from build123d import *

# Parameters (mm, degrees)
SKETCH1_W                  = 231.4
SKETCH1_H                  = 30
BOSS_EXTRUDE1_DEPTH        = 3
BOSS_EXTRUDE2_DEPTH        = 3
F_8_0_8_DIAMETER_HOLE1_D   = 8
F_8_0_8_DIAMETER_HOLE2_D   = 8
F_10_0_10_DIAMETER_HOLE1_D = 10


with BuildPart() as part:
    # Sketch1 → Boss-Extrude1 (new body)
    with BuildSketch(Plane.XY):
        with Locations((0, -15)):
            Rectangle(SKETCH1_W, SKETCH1_H)
    extrude(amount=BOSS_EXTRUDE1_DEPTH)

    # Sketch2 → Boss-Extrude2 (add)
    with BuildSketch(Plane(origin=(0, 0, 0), x_dir=(1, 0, 0), z_dir=(0, 1, 0))):
        Polygon((-115.7, -3), (115.7, -3), (85.7, -33), (-85.7, -33), align=None)
    extrude(amount=-BOSS_EXTRUDE2_DEPTH)

    # Ø8.0 (8) Diameter Hole1 (through all)
    with Locations(Plane.XY.offset(3)):
        with Locations((-100.7, -15), (100.7, -15)):
            Hole(F_8_0_8_DIAMETER_HOLE1_D / 2)

    # Ø8.0 (8) Diameter Hole2 (through all)
    with Locations(Plane(origin=(0, 0, 0), x_dir=(1, 0, 0), z_dir=(0, 1, 0))):
        with Locations((0, -18)):
            Hole(F_8_0_8_DIAMETER_HOLE2_D / 2)

    # Ø10.0 (10) Diameter Hole1 (through all)
    with Locations(Plane.XY.offset(3)):
        with Locations((62.5, -15)):
            Hole(F_10_0_10_DIAMETER_HOLE1_D / 2)


solid = part.part
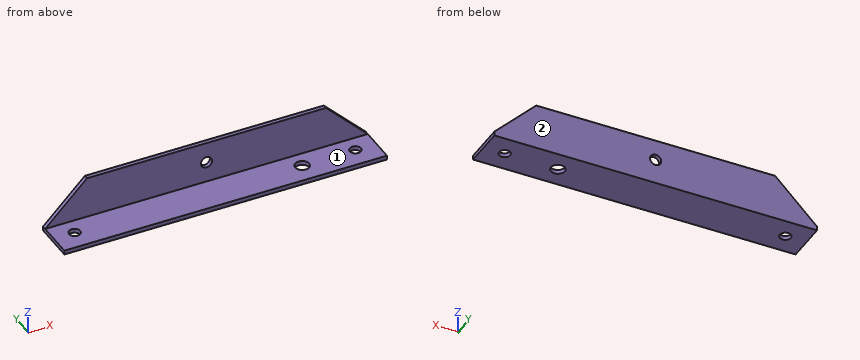
Here's how the part is built. I have some questions about the finished solid (model axes, mm). Face numbers are marked on the shaded views. A direction names the side the tool comes from. Coordinates: 2 decimals unless noted, no trailing zeros. Write each loop counter-clockwise with the first axis right and the second up, starting at its lowest first coordinate (ties: lowest second). Pieces come first, ordered by that corner, then holes.
1) I'm going to push flat-ended pins straight in: pin 1 (3 mm diameter, centred on x = -5.5, y = -16.5, fed in from +Z); pin 2 (10 mm diameter, centred on y = -10.5, z = 25.5, fed in from +X); pin 3 (15 mm diameter, centred on x = -5.5, z = 25.5, fed in from -Y). Where does each tip first touch, or does it pass through?
Filled in:
pin 1: stops at z = 3
pin 2: passes through
pin 3: stops at y = -3
2) If we section it at B-B (y = -15): List the corners of the cut face in (x, z) for me, plus the area to 3 significant figures.
Filled in:
outline: (-115.7, 0) - (-104.7, 0) - (-104.7, 3) - (-115.7, 3) - close; (-96.7, 0) - (57.5, 0) - (57.5, 3) - (-96.7, 3) - close; (67.5, 0) - (96.7, 0) - (96.7, 3) - (67.5, 3) - close; (104.7, 0) - (115.7, 0) - (115.7, 3) - (104.7, 3) - close
area: 616 mm2
3) If we section it at C-C (z = 18): List the corners of the cut face in (x, y) for me.
Filled in:
outline: (-100.7, -3) - (-4, -3) - (-4, 0) - (-100.7, 0) - close; (4, -3) - (100.7, -3) - (100.7, 0) - (4, 0) - close
4) Which directions (+Z, -Z, +X, -X, +Y, -Y) give clear straight access to the entire face, cutting with the end or side of a thin tool? Please do the marked faces 1 and 2.
Filled in:
face 1: +Z, +X, -X, -Y
face 2: +Z, -Z, +X, -X, +Y
5) If we section it at D-D (x = 0): List the corners of the cut face in (y, z) for me.
Filled in:
outline: (-30, 0) - (0, 0) - (0, 14) - (-3, 14) - (-3, 3) - (-30, 3) - close; (-3, 22) - (0, 22) - (0, 33) - (-3, 33) - close
6) If I drill on line 1 (Y direction, x = -100.7, z = 0.6); line 2 (Z direction, x = 0, y = -2.25); line 3 (Z direction, x = -24.5, y = -21.5), over which ranges is the centre line in solid material (lowest first)?
Filled in:
line 1: y = -30 to -19, -11 to 0
line 2: z = 0 to 14, 22 to 33
line 3: z = 0 to 3
7) If we section it at A-A (x = -100.7): List the corners of the cut face in (y, z) for me, plus the area to 3 significant figures.
Filled in:
outline: (-30, 0) - (-19, 0) - (-19, 3) - (-30, 3) - close; (-11, 0) - (0, 0) - (0, 18) - (-3, 18) - (-3, 3) - (-11, 3) - close
area: 111 mm2
